Could you check a few things on this drawing? It's one solid part, dimensions in mm from its lowest x, y, z. Give positions to 0.01 mm unless a question says otherwise; leave off trailing zeros. Write each loop counter-clockwise with the first axis right and the second up, starting at its lowest first coordinate (ties: lowest second). Pieces come first, ordered by that corner, then holes. Notation, with made-up numbers: M -32.5,88 L 9.5,88 A23 ccw 9.5,107 Z; hole C 23,-3 d2. An arc over 180 degrees is marked long. Write each question's results on one line, items separated by ' | '.
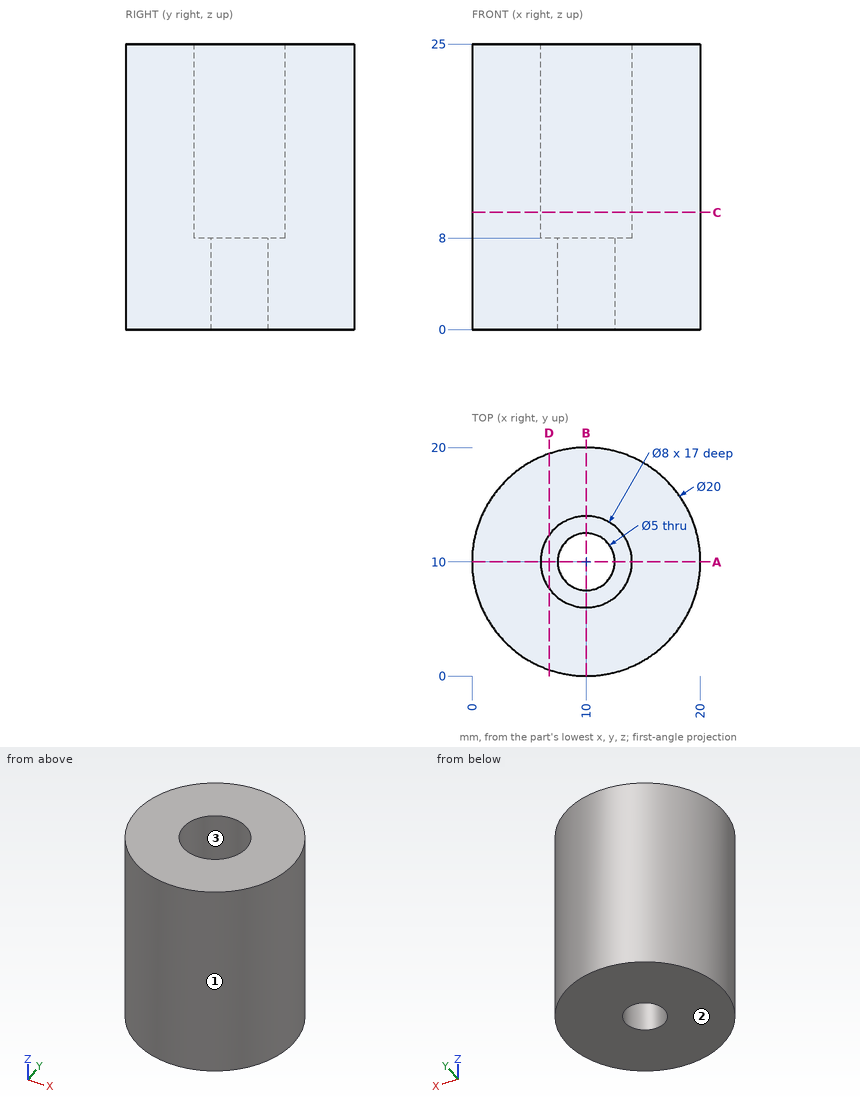
Item 1: I want a section at C-C, the plane z = 10.25. Please give me the cut outline in (x, y), and give its area (3 significant figures).
Geometry says:
outline: C 10,10 d20; hole C 10,10 d8 | area: 264 mm2
Item 2: Thinking about a two-plate mould opening in Y: for the marked faces 1, 2 and 3, which applies, +Y half, -Y half, draft (parallel to the pull), parting line (faces both ways), or undercut?
Geometry says:
face 1: parting line | face 2: draft | face 3: undercut
Item 3: I want a section at D-D, the plane x = 6.75. Please give me the cut outline in (y, z).
Geometry says:
outline: M 0.54,0 L 19.46,0 L 19.46,25 L 12.33,25 L 12.33,8 L 7.67,8 L 7.67,25 L 0.54,25 Z
Item 4: I'm going to push flat-ended pins straight in: pin 1 (2.5 mm diameter, centred on x = 8.5, y = 10.5, fed in from +Z); pin 2 (4 mm diameter, centred on x = 3.5, z = 14.5, fed in from +Y); pin 3 (3 mm diameter, centred on y = 15, z = 15.5, fed in from -X). Where does each tip first touch, or does it pass through?
Geometry says:
pin 1: stops at z = 8 | pin 2: stops at y = 18.93 | pin 3: stops at x = 0.63
Item 5: I want a section at A-A, the plane y = 10. Please give me the cut outline in (x, z), and give its area (3 significant figures).
Geometry says:
outline: M 0,0 L 7.5,0 L 7.5,8 L 6,8 L 6,25 L 0,25 Z; M 12.5,0 L 20,0 L 20,25 L 14,25 L 14,8 L 12.5,8 Z | area: 324 mm2
Item 6: If I drill on line 1 (Y direction, x = 10, z = 3.25); line 2 (Y direction, x = 10, z = 18.75); line 3 (X direction, y = 9, z = 16), over which ranges is the centre line in solid material (lowest first)? Write a range as from..to.
Geometry says:
line 1: y = 0..7.5, 12.5..20 | line 2: y = 0..6, 14..20 | line 3: x = 0.05..6.13, 13.87..19.95
